```python
from build123d import *

# Parameters (mm, degrees)
F0_W     = 151.962713
F0_H     = 151.340999
F1_DEPTH = 25.4
F2_R     = 31.640714
F3_DEPTH = 50.8
F5_DEPTH = 74.422


with BuildPart() as f1:
    # F0 (on Top) → F1 (new body)
    with BuildSketch(Plane.XY):
        with Locations((-0.302956, 0.808675)):
            Rectangle(F0_W, F0_H)
    extrude(amount=F1_DEPTH)

    # F2 (on face) → F3 (join)
    with BuildSketch(Plane.XY.offset(25.4)):
        Circle(F2_R)
    extrude(amount=F3_DEPTH)

    # F4 (on Right) → F5 (cut, symmetric)
    with BuildSketch(Plane.YZ):
        Polygon((52.56303, 76.373637), (-43.877404, 76.373637), (52.56303, 45.524683), align=None)
    extrude(amount=F5_DEPTH, both=True, mode=Mode.SUBTRACT)


solid = f1.part
```
Geometry check sheet. Reference: the model listing, model coordinates, mm. A direction names the side the tool comes from. Round coordinates to 2 decimals unless told otherwise and drop trailing zeros. Order: outer loops, then holes, each group sorted by start corner. A loop starts at its lowest first (then second) coordinate and runs counter-clockwise, first axis right, second up. Notation, with made-up numbers: (64, -38.5) - (83, -38.5) arc R20 ccw to (83, -1.5) - close; hole circle Ø4 at (50, 6). An arc over 180 degrees is marked (long way). Use a Markdown table: item, result. Add a question column.
1) Set-up check for faces 1 (the cylindrical face through (-6.86, -30.89, 43.37)), 2 (the flat face through (0.44, -0.44, 62.48)): record each of +Z, -Z, +X, -X, +Y, -Y from which the full face is reachable in a straight line by a thin tool's end or side.
2) Section check D-D (x = -44.5). Record the cut outline in (y, z).
3) Gauge pin test, flat ends, axial feed: P1, Ø6, axis at y = 5, z = 30.5, coming from the -X side; P2, Ø1.5, axis at x = -40.5, y = -38, coming from the +Z side; P3, Ø4, axis at y = 3.5, z = 29, coming from the +X side. Record the tip position at first contact, or that the pin passes through.
4) Section check B-B (z = 37). Record the cut outline in (x, y), then the cut area to 3 significant figures.
5) Section check A-A (x = 0). Record the cut outline in (y, z).
6) Section check C-C (y = -52). Record the cut outline in (x, z).
7) Thickness scan on line 1 along Z through (x, y) = (5, -45); line 2 along X through (y, z) = (19, 32); line 3 along Z through (x, y) = (9, -21). Record the ranges inside material, lowest first.
Established:
| question | item | result |
|---|---|---|
| 1 | face 1 | +Z |
| 1 | face 2 | +Z, +X, -X, +Y |
| 2 | outline | (-74.86, 0) - (76.48, 0) - (76.48, 25.4) - (-74.86, 25.4) - close |
| 3 | P1 | x = -31.58 |
| 3 | P2 | z = 25.4 |
| 3 | P3 | x = 31.61 |
| 4 | outline | circle Ø63.28 at (0, 0) |
| 4 | area | 3,150 mm2 |
| 5 | outline | (-74.86, 0) - (76.48, 0) - (76.48, 25.4) - (31.64, 25.4) - (31.64, 52.22) - (-31.64, 72.46) - (-31.64, 25.4) - (-74.86, 25.4) - close |
| 6 | outline | (-76.28, 0) - (75.68, 0) - (75.68, 25.4) - (-76.28, 25.4) - close |
| 7 | line 1 | 0 to 25.4 |
| 7 | line 2 | -25.3 to 25.3 |
| 7 | line 3 | 0 to 69.06 |
